Part model, mm, in its own coordinate system. Face numbers are marked on the shaded views. A direction names the side the tool comes from. Coordinates: 2 decimals unless noted, no trailing zeros. Loops run counter-clockwise (first coordinate to the right, second up) from the corner with the lowest first, then second, coordinate; pieces in that order, holes last. Notation, with made-up numbers: (-25, 58) - (6, 58) arc R21 cw to (6, 92) - close; hole circle Ø6 at (-19.75, -8.5). An arc over 180 degrees is marked (long way). Use a Markdown table: item, result. Add a question column.
1) Band-saw the part on B-B (y = 0). Give the cut face in (x, z).
2) Drop flat-ended pins along their axis: P1, Ø2, axis at x = -19, z = 0.5, coming from the -Y side; P2, Ø0.8, axis at x = -6.5, z = 3.5, coming from the +Y side; P3, Ø3, axis at y = 2, z = 2.5, coming from the +X side. Give the stop position or say it passes through.
3) Band-saw the part on C-C (x = 13). Give the cut face in (y, z).
4) Band-saw the part on A-A (z = 1.5). Give the cut face in (x, y), plus the area to 3 significant figures.
5) Band-saw the part on D-D (y = -3.25). Give the cut face in (x, z), plus the area to 3 significant figures.
6) Tool access for the marked faces 1, 2 and 3: list every direction of +Z, -Z, +X, -X, +Y, -Y with a clear straight run to the whole face (end or side of a thin tool).
7) Probe probe 1 along Y at (x, z) = (-5, 2.15); probe 2 along X at (y, z) = (-0.25, 0.8); probe 3 along Y at (x, z) = (23, 3.7). List the from-to ranges inside material, lowest first. Write a range as [from, to].
from build123d import *

# Parameters (mm, degrees)
SKETCH_W        = 61
SKETCH_H        = 16.5
PAD_DEPTH       = 6
SKETCH001_W     = 55
SKETCH001_H     = 10.5
SKETCH001_R     = 1
POCKET_DEPTH    = 3
SKETCH002_W     = 55
SKETCH002_H     = 6
POCKET001_DEPTH = 4
PAD001_START    = 5
SKETCH003_W     = 81
SKETCH003_H     = 22.5
SKETCH003_R     = 2
PAD001_DEPTH    = 1
FILLET_R        = 5


with BuildPart() as part:
    # Sketch → Pad (new body)
    with BuildSketch(Plane.XY):
        Rectangle(SKETCH_W, SKETCH_H)
    extrude(amount=PAD_DEPTH)

    # Sketch001 → Pocket (cut)
    with BuildSketch(Plane.XY):
        Rectangle(SKETCH001_W, SKETCH001_H)
        with Locations((-13, -3.25)):
            Circle(SKETCH001_R, mode=Mode.SUBTRACT)
        with Locations((13, -3.25)):
            Circle(SKETCH001_R, mode=Mode.SUBTRACT)
    extrude(amount=POCKET_DEPTH, mode=Mode.SUBTRACT)

    # Sketch002 → Pocket001 (cut)
    with BuildSketch(Plane.XY):
        with Locations((0, 2.25)):
            Rectangle(SKETCH002_W, SKETCH002_H)
    extrude(amount=POCKET001_DEPTH, mode=Mode.SUBTRACT)

    # Sketch003 → Pad001 (join)
    with BuildSketch(Plane.XY.offset(PAD001_START)):
        Rectangle(SKETCH003_W, SKETCH003_H)
        with Locations((36.5, 0)):
            Circle(SKETCH003_R, mode=Mode.SUBTRACT)
        with Locations((-36.5, 0)):
            Circle(SKETCH003_R, mode=Mode.SUBTRACT)
    extrude(amount=PAD001_DEPTH)

    # Fillet
    fillet_edges = [part.edges().sort_by_distance(p)[0] for p in [
        (-40.5, 11.25, 5.5),
        (-40.5, -11.25, 5.5),
        (40.5, -11.25, 5.5),
        (40.5, 11.25, 5.5),
    ]]
    fillet(fillet_edges, radius=FILLET_R)


solid = part.part
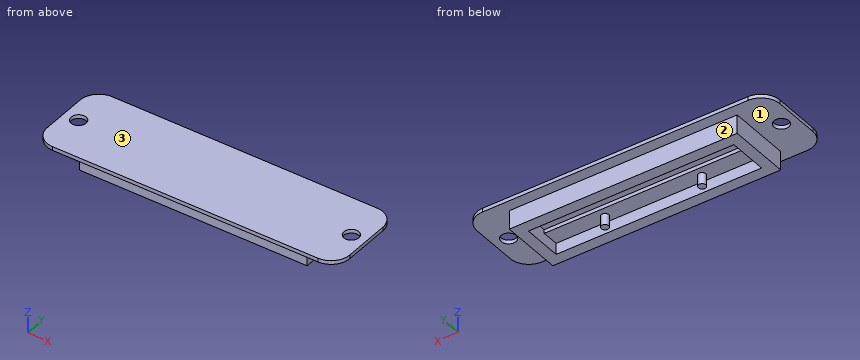
Answer block:
| question | item | result |
|---|---|---|
| 1 | outline | (-40.5, 5) - (-38.5, 5) - (-38.5, 6) - (-40.5, 6) - close; (-34.5, 5) - (-30.5, 5) - (-30.5, 0) - (-27.5, 0) - (-27.5, 4) - (27.5, 4) - (27.5, 0) - (30.5, 0) - (30.5, 5) - (34.5, 5) - (34.5, 6) - (-34.5, 6) - close; (38.5, 5) - (40.5, 5) - (40.5, 6) - (38.5, 6) - close |
| 2 | P1 | y = -8.25 |
| 2 | P2 | y = 8.25 |
| 2 | P3 | x = 30.5 |
| 3 | outline | (-11.25, 5) - (-8.25, 5) - (-8.25, 0) - (-5.25, 0) - (-5.25, 3) - (-4.25, 3) - (-4.25, 0) - (-2.25, 0) - (-2.25, 3) - (-0.75, 3) - (-0.75, 4) - (5.25, 4) - (5.25, 0) - (8.25, 0) - (8.25, 5) - (11.25, 5) - (11.25, 6) - (-11.25, 6) - close |
| 4 | outline | (-30.5, -8.25) - (30.5, -8.25) - (30.5, 8.25) - (-30.5, 8.25) - close; circle Ø2 at (-13, -3.25); circle Ø2 at (13, -3.25); hole (-27.5, -5.25) - (27.5, -5.25) - (27.5, 5.25) - (-27.5, 5.25) - close |
| 4 | area | 435 mm2 |
| 5 | outline | (-40.5, 5) - (-30.5, 5) - (-30.5, 0) - (-27.5, 0) - (-27.5, 3) - (-14, 3) - (-14, 0) - (-12, 0) - (-12, 3) - (12, 3) - (12, 0) - (14, 0) - (14, 3) - (27.5, 3) - (27.5, 0) - (30.5, 0) - (30.5, 5) - (40.5, 5) - (40.5, 6) - (-40.5, 6) - close |
| 5 | area | 233 mm2 |
| 6 | face 1 | -Z |
| 6 | face 2 | -Z, +X, -X, +Y |
| 6 | face 3 | +Z, +X, -X, +Y, -Y |
| 7 | probe 1 | [-8.25, -5.25], [5.25, 8.25] |
| 7 | probe 2 | [-30.5, -27.5], [27.5, 30.5] |
| 7 | probe 3 | [-8.25, -0.75], [5.25, 8.25] |
